Verification items for the finished model (mm, model axes). Face numbers are marked on the shaded views. Give positions to 0.01 mm unless a question says otherwise; leave off trailing zeros. Order: outer loops, then holes, each group sorted by start corner. A loop starts at its lowest first (then second) coordinate and runs counter-clockwise, first axis right, second up.
(1) Sectioned sample at B-B on z = 0.6. Record the cut outline in (x, y) (3 decimals).
(2) Gauge pin test, flat ends, axial feed: pin 1 (0.5 mm diameter, centred on x = 0, z = -0.5, fed in from -Y); pin 2 (0.6 mm diameter, centred on y = 2.5, z = -0.5, fed in from +X) (3 decimals); pin 3 (0.6 mm diameter, centred on y = 2.5, z = -0.5, fed in from -X) (3 decimals). Record the tip position at first contact, or that the pin passes through.
(3) Scan lines: L1, parallel to Y at x = -1.6, z = 0.05; L2, parallel to Z at x = -2.2, y = 1; L3, parallel to Z at x = -0.2, y = -1.9. Record each from-to range of solid material in increasing order.
(4) Mould release check, pull along Y, two halves, no side actions. Record for the marked faces 1 and 2: pulls with the +Y half, pulls with the -Y half, needs draft (parallel to the pull), parting line crosses it, or undercut.
(5) Sectioned sample at C-C on y = -0.05. Record the cut outline in (x, z) (3 decimals), plus the area to 4 significant figures.
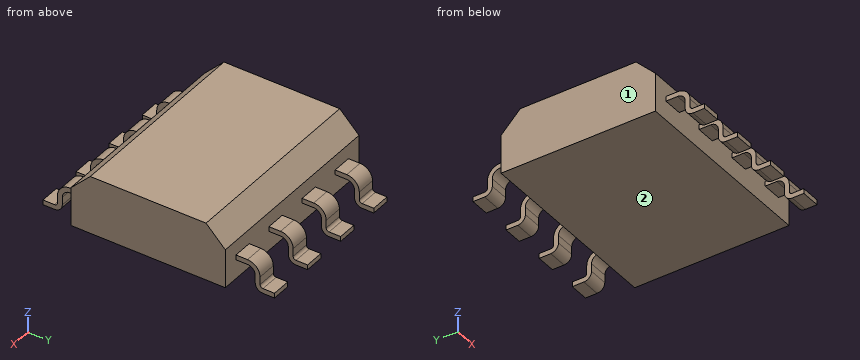
```python
from build123d import *

# Parameters (mm, degrees)
SKETCH1_W               = 5.05
SKETCH1_H               = 4
EXTRUDE1_DEPTH          = 0.75
CHAMFER1_SIZE           = 0.5
SKETCH2_W               = 0.5
SKETCH2_H               = 0.125
LPATTERN1_COUNT         = 4
LPATTERN1_PITCH         = 1.25
MIRROR1_COPY_1_SKETCH_W = 0.5
MIRROR1_COPY_1_SKETCH_H = 0.125
MIRROR1_COPY_2_SKETCH_W = 0.5
MIRROR1_COPY_2_SKETCH_H = 0.125
MIRROR1_COPY_3_SKETCH_W = 0.5
MIRROR1_COPY_3_SKETCH_H = 0.125


with BuildPart() as part:
    # Sketch1 → Extrude1 (new, symmetric)
    with BuildSketch(Plane.XY):
        Rectangle(SKETCH1_W, SKETCH1_H)
    extrude(amount=EXTRUDE1_DEPTH, both=True)

    # Chamfer1
    chamfer1_edges = [part.edges().sort_by_distance(p)[0] for p in [
        (0, -2, 0.75),
        (0, 2, 0.75),
    ]]
    chamfer(chamfer1_edges, length=CHAMFER1_SIZE)

    # Sweep1: sweep along a path in Sketch3
    with BuildLine(Plane(origin=(2.125, 0, 0), x_dir=(0, 0, -1), z_dir=(1, 0, 0))) as sweep1_path:
        Line((0.85, 3), (0.85, 2.7))
        ThreePointArc((0.85, 2.7), (0.791421356, 2.558578644), (0.65, 2.5))
        Line((0.65, 2.5), (0.45, 2.5))
        ThreePointArc((0.45, 2.5), (0.308578644, 2.441421356), (0.25, 2.3))
        Line((0.25, 2.3), (0.25, 2))
    # Sketch2 → Sweep1 (sweep)
    with BuildSketch(Plane(origin=(0, 2, 0), x_dir=(1, 0, 0), z_dir=(0, 1, 0))):
        with Locations((1.875, 0.1875)):
            Rectangle(SKETCH2_W, SKETCH2_H)
    sweep1 = sweep(path=sweep1_path.line)

    # LPattern1: Sweep1 ×4
    with Locations(*[(-i * LPATTERN1_PITCH, 0, 0) for i in range(1, LPATTERN1_COUNT)]):
        add(sweep1)

    # Mirror1: Sweep1 across plane
    add(sweep1.mirror(Plane.ZX))

    # Mirror1 copy 1: sweep along a path in Mirror1 copy 1 path
    with BuildLine(Plane(origin=(0.875, 0, 0), x_dir=(0, 0, -1), z_dir=(1, 0, 0))) as mirror1_copy_1_path:
        Line((0.85, -3), (0.85, -2.7))
        ThreePointArc((0.85, -2.7), (0.791421356, -2.558578644), (0.65, -2.5))
        Line((0.65, -2.5), (0.45, -2.5))
        ThreePointArc((0.45, -2.5), (0.308578644, -2.441421356), (0.25, -2.3))
        Line((0.25, -2.3), (0.25, -2))
    # Mirror1 copy 1 sketch → Mirror1 copy 1 (sweep)
    with BuildSketch(Plane(origin=(-1.25, -2, 0), x_dir=(1, 0, 0), z_dir=(0, -1, 0))):
        with Locations((1.875, -0.1875)):
            Rectangle(MIRROR1_COPY_1_SKETCH_W, MIRROR1_COPY_1_SKETCH_H)
    sweep(path=mirror1_copy_1_path.line)

    # Mirror1 copy 2: sweep along a path in Mirror1 copy 2 path
    with BuildLine(Plane(origin=(-0.375, 0, 0), x_dir=(0, 0, -1), z_dir=(1, 0, 0))) as mirror1_copy_2_path:
        Line((0.85, -3), (0.85, -2.7))
        ThreePointArc((0.85, -2.7), (0.791421356, -2.558578644), (0.65, -2.5))
        Line((0.65, -2.5), (0.45, -2.5))
        ThreePointArc((0.45, -2.5), (0.308578644, -2.441421356), (0.25, -2.3))
        Line((0.25, -2.3), (0.25, -2))
    # Mirror1 copy 2 sketch → Mirror1 copy 2 (sweep)
    with BuildSketch(Plane(origin=(-2.5, -2, 0), x_dir=(1, 0, 0), z_dir=(0, -1, 0))):
        with Locations((1.875, -0.1875)):
            Rectangle(MIRROR1_COPY_2_SKETCH_W, MIRROR1_COPY_2_SKETCH_H)
    sweep(path=mirror1_copy_2_path.line)

    # Mirror1 copy 3: sweep along a path in Mirror1 copy 3 path
    with BuildLine(Plane(origin=(-1.625, 0, 0), x_dir=(0, 0, -1), z_dir=(1, 0, 0))) as mirror1_copy_3_path:
        Line((0.85, -3), (0.85, -2.7))
        ThreePointArc((0.85, -2.7), (0.791421356, -2.558578644), (0.65, -2.5))
        Line((0.65, -2.5), (0.45, -2.5))
        ThreePointArc((0.45, -2.5), (0.308578644, -2.441421356), (0.25, -2.3))
        Line((0.25, -2.3), (0.25, -2))
    # Mirror1 copy 3 sketch → Mirror1 copy 3 (sweep)
    with BuildSketch(Plane(origin=(-3.75, -2, 0), x_dir=(1, 0, 0), z_dir=(0, -1, 0))):
        with Locations((1.875, -0.1875)):
            Rectangle(MIRROR1_COPY_3_SKETCH_W, MIRROR1_COPY_3_SKETCH_H)
    sweep(path=mirror1_copy_3_path.line)


solid = part.part
```
Ans:
1. outline: (-2.525, -1.65) - (2.525, -1.65) - (2.525, 1.65) - (-2.525, 1.65) - close
2. pin 1: stops at y = -2
2. pin 2: stops at x = 2.125
2. pin 3: stops at x = -2.125
3. L1: y = -2 to 2
3. L2: z = -0.75 to 0.75
3. L3: z = -0.75 to 0.35
4. face 1: needs draft
4. face 2: undercut
5. outline: (-2.525, -0.75) - (2.525, -0.75) - (2.525, 0.75) - (-2.525, 0.75) - close
5. area: 7.575 mm2
